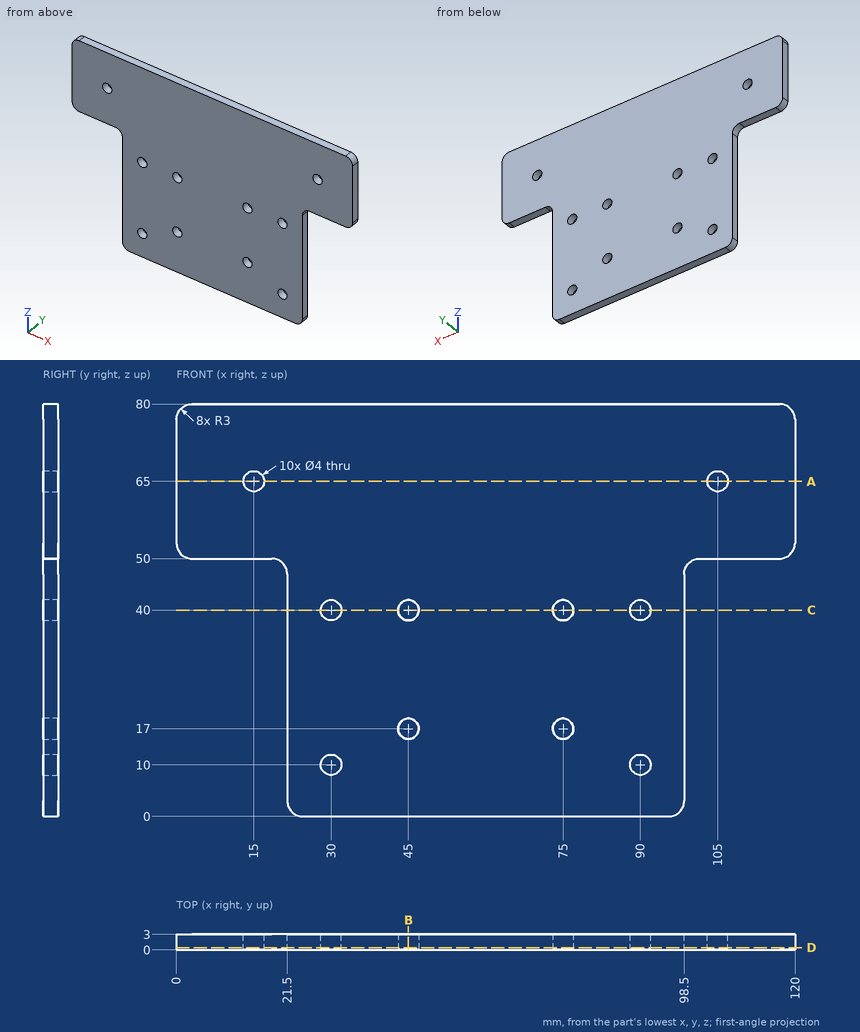
Design review of the part shown in the three views and the two pictorial views. Dimensions are in mm from the part's minimum x, y and z. Round coordinates to 2 decimals unless told otherwise and drop trailing zeros. Loops run counter-clockwise (first coordinate to the right, second up) from the corner with the lowest first, then second, coordinate; pieces in that order, holes last.
(1) We need section B-B (x = 45). Give the boundary of the cut face in (y, z), plus the area to 3 significant figures.
Returned:
outline: (0, 0) - (3, 0) - (3, 15) - (0, 15) - close; (0, 19) - (3, 19) - (3, 38) - (0, 38) - close; (0, 42) - (3, 42) - (3, 80) - (0, 80) - close
area: 216 mm2
(2) We need section C-C (z = 40). Give the boundary of the cut face in (x, y).
Returned:
outline: (21.5, 0) - (28, 0) - (28, 3) - (21.5, 3) - close; (32, 0) - (43, 0) - (43, 3) - (32, 3) - close; (47, 0) - (73, 0) - (73, 3) - (47, 3) - close; (77, 0) - (88, 0) - (88, 3) - (77, 3) - close; (92, 0) - (98.5, 0) - (98.5, 3) - (92, 3) - close
(3) Clearance check with flat-ended pins moving along their axes: P1, Ø3.5, axis at x = 105, z = 65, coming from the -Y side; P2, Ø1.5, axis at x = 7.5, y = 1, coming from the -Z side; P3, Ø1.5, axis at y = 1.5, z = 19, coming from the +X side. State where each tip first meets the part, or that it passes through.
Returned:
P1: passes through
P2: stops at z = 50
P3: stops at x = 98.5
(4) We need section D-D (y = 0.45). State how many separate pieces and enclosed holes the cut face has, plus the area to 3 significant figures.
Returned:
separate pieces: 1
enclosed holes: 10
area: 7,320 mm2
(5) We need section A-A (z = 65). Give the boundary of the cut face in (x, y), plus the area to 3 significant figures.
Returned:
outline: (0, 0) - (13, 0) - (13, 3) - (0, 3) - close; (17, 0) - (103, 0) - (103, 3) - (17, 3) - close; (107, 0) - (120, 0) - (120, 3) - (107, 3) - close
area: 336 mm2
(6) Wall thickness on line 1 along X through (y, z) = (2.25, 40); line 2 along Z through (x, y) = (45, 1.2); line 3 along Z through (x, y) = (90, 1): over which ranges is each line inside the solid? List them lowest first.
Returned:
line 1: x = 21.5 to 28, 32 to 43, 47 to 73, 77 to 88, 92 to 98.5
line 2: z = 0 to 15, 19 to 38, 42 to 80
line 3: z = 0 to 8, 12 to 38, 42 to 80
